```python
from build123d import *

# Parameters (mm, degrees)
SKETCH1_W           = 9.4
SKETCH1_H           = 2
BOSS_EXTRUDE1_DEPTH = 85.5
BOSS_EXTRUDE2_DEPTH = 81
FILLET1_R           = 0.5
BOSS_EXTRUDE3_DEPTH = 78
SKETCH2_R           = 1.5
CUT_EXTRUDE1_DEPTH  = 87.643786319
CUT_EXTRUDE2_REACH  = 88.644
SKETCH2_3_W         = 4.8
SKETCH2_3_H         = 4
SKETCH2_3_W_2       = 2.2
SKETCH3_W           = 2
SKETCH3_H           = 63
CUT_EXTRUDE3_DEPTH  = 5
SKETCH4_W           = 1
SKETCH4_H           = 3.5
CUT_EXTRUDE4_DEPTH  = 2


with BuildPart() as part:
    # Sketch1 → Boss-Extrude1 (new body)
    with BuildSketch(Plane(origin=(0, 0, 0), x_dir=(1, 0, 0), z_dir=(0, 1, 0))):
        with Locations((0.278560628, 2.818575451)):
            Rectangle(SKETCH1_W, SKETCH1_H)
    extrude(amount=-BOSS_EXTRUDE1_DEPTH)

    # Sketch1<3> → Boss-Extrude2 (add)
    with BuildSketch(Plane(origin=(0, 0, 0), x_dir=(1, 0, 0), z_dir=(0, 1, 0))):
        Polygon((3.978560628, 1.818575451), (-3.421439372, 1.818575451), (-3.421439372, 0.818575451), (-4.421439372, 0.818575451), (-4.421439372, -0.181424549), (4.978560628, -0.181424549), (4.978560628, 0.818575451), (3.978560628, 0.818575451), align=None)
    extrude(amount=-BOSS_EXTRUDE2_DEPTH)

    # Fillet1
    fillet1_edges = [part.edges().sort_by_distance(p)[0] for p in [
        (-4.421439372, -85.5, -2.818575451),
        (4.978560628, -85.5, -2.818575451),
        (-4.421439372, 0, -2.818575451),
        (0.278560628, 0, -3.818575451),
        (4.978560628, 0, -2.818575451),
        (-4.421439372, -42.75, -3.818575451),
        (4.978560628, -42.75, -3.818575451),
        (0.278560628, -85.5, -3.818575451),
    ]]
    fillet(fillet1_edges, radius=FILLET1_R)

    # Sketch1<4> → Boss-Extrude3 (add)
    with BuildSketch(Plane(origin=(0, 0, 0), x_dir=(1, 0, 0), z_dir=(0, 1, 0))):
        Polygon((-5.421439372, -0.181424549), (-4.421439372, -0.181424549), (4.978560628, -0.181424549), (5.978560628, -0.181424549), (5.978560628, -8.181424549), (2.978560628, -8.181424549), (2.978560628, -3.181424549), (-4.050977977, -3.181424549), (-4.050977977, -1.181424549), (-5.421439372, -1.181424549), align=None)
    extrude(amount=-BOSS_EXTRUDE3_DEPTH)

    # Sketch2 → Cut-Extrude1 (cut, through all)
    with BuildSketch(Plane(origin=(5.978560628, 0, 0), x_dir=(0, 0, -1), z_dir=(1, 0, 0))):
        with Locations((-5.681424549, -12.5)):
            Circle(SKETCH2_R)
        with Locations((-4.181424549, -75)):
            Circle(SKETCH2_R)
    extrude(amount=-CUT_EXTRUDE1_DEPTH, mode=Mode.SUBTRACT)

    # Cut-Extrude2: up to this face of the body (flat: up to its plane)
    cut_extrude2_end = Plane(part.part.faces().sort_by_distance((3.978560628, -40.5, -1.318575451))[0])
    # Sketch2<3> → Cut-Extrude2 (cut, up to the picked face)
    with BuildSketch(Plane(origin=(5.978560628, 0, 0), x_dir=(0, 0, -1), z_dir=(1, 0, 0)), mode=Mode.PRIVATE) as cut_extrude2_sk1:
        with Locations((-2.581424549, -7)):
            Rectangle(SKETCH2_3_W, SKETCH2_3_H)
    cut_extrude2_tool1 = split(extrude(cut_extrude2_sk1.sketch, amount=-CUT_EXTRUDE2_REACH, mode=Mode.PRIVATE), bisect_by=cut_extrude2_end, keep=Keep.BOTH, mode=Mode.PRIVATE)
    # Sketch2<3> → Cut-Extrude2 (cut, up to the picked face)
    with BuildSketch(Plane(origin=(5.978560628, 0, 0), x_dir=(0, 0, -1), z_dir=(1, 0, 0)), mode=Mode.PRIVATE) as cut_extrude2_sk2:
        with Locations((0.918575451, -7)):
            Rectangle(SKETCH2_3_W_2, SKETCH2_3_H)
    cut_extrude2_tool2 = split(extrude(cut_extrude2_sk2.sketch, amount=-CUT_EXTRUDE2_REACH, mode=Mode.PRIVATE), bisect_by=cut_extrude2_end, keep=Keep.BOTH, mode=Mode.PRIVATE)
    add(cut_extrude2_tool1.solids().sort_by(Axis((5.978561, -7, 2.581425), (-1, 0, 0)))[0], mode=Mode.SUBTRACT)
    add(cut_extrude2_tool2.solids().sort_by(Axis((5.978561, -7, -0.918575), (-1, 0, 0)))[0], mode=Mode.SUBTRACT)

    # Sketch3 → Cut-Extrude3 (cut)
    with BuildSketch(Plane.XY.offset(8.181424549)):
        with Locations((3.978560628, -46.5)):
            Rectangle(SKETCH3_W, SKETCH3_H)
    extrude(amount=-CUT_EXTRUDE3_DEPTH, mode=Mode.SUBTRACT)

    # Sketch4 → Cut-Extrude4 (cut)
    with BuildSketch(Plane(origin=(5.978560628, 0, 0), x_dir=(0, 0, -1), z_dir=(1, 0, 0))):
        with Locations((-2.681424549, -26.75)):
            Rectangle(SKETCH4_W, SKETCH4_H)
        with Locations((-2.681424549, -56.25)):
            Rectangle(SKETCH4_W, SKETCH4_H)
    extrude(amount=-CUT_EXTRUDE4_DEPTH, mode=Mode.SUBTRACT)


with BuildPart() as body_2:
    # Mirror1: mirrored copy
    add(part.part.mirror(Plane(origin=(0, 0, -13.818575451), x_dir=(1, 0, 0), z_dir=(0, 0, -1))))


solid = body_2.part
```
Part model, mm, in its own coordinate system. A direction names the side the tool comes from. Round coordinates to 2 decimals unless told otherwise and drop trailing zeros. Order: outer loops, then holes, each group sorted by start corner. A loop starts at its lowest first (then second) coordinate and runs counter-clockwise, first axis right, second up. Notation, with made-up numbers: M 65,27 L 72,27 A37 cw 72,64 Z; hole C -16,7.25 d8. An arc over 180 degrees is marked long. Answer in a Markdown table with one row per item. Add a question column.
Q1. Wall check: L1, parallel to Z at x = -4, y = -9.5; L2, parallel to Y at x = 1.5, z = -29.5; L3, parallel to X at y = -53, z = -34. Give the ranges that are in metal, low to high. Write a range as from..to.
Q2. Cut at C-C on y = -63.5. Give the cut face in (x, z).
Q3. Cut at A-A on y = -12.5. Give the cut face in (x, z).
Q4. 3-axis set-ups, long thin cutter, end or side, ignore diameter. For faces 5 (the face through (4, -15, -33)), 6 (the face through (-4, -52, -25.819)), 7 (the face through (0, -79, -27.819)): which of +Z, -Z, +X, -X, +Y, -Y reach the whole face in a straight line?
Q5. Pin check, flat tips, straight feed: pin 1 (0.8 mm diameter, centred on y = -55, z = -25, fed in from -X); pin 2 (0.8 mm diameter, centred on x = 5.5, y = -55.5, fed in from +Z); pin 3 (0.5 mm diameter, centred on x = 5.5, z = -30.5, fed in from -Y). Stop position of each tip, or through.
Q6. Mould opens along Z. For faces 1 (the face through (5, -7, -32.619)), 2 (the face through (1, -77, -30.819)), 3 (the face through (0, -42, -23.819)), 4 (the face through (-4.421, -42, -25)) say: +Z half, -Z half, draft (parallel to the pull), parting line (faces both ways), or undercut.
Q7. Cut at B-B on x = 1.5. Give the cut face in (y, z).
Established:
| question | item | result |
|---|---|---|
| 1 | L1 | z = -30.82..-26.82, -25.82..-23.82 |
| 1 | L2 | y = -78..0 |
| 1 | L3 | x = 4.98..5.98 |
| 2 | outline | M -5.42,-28.82 L -4.05,-28.82 L -4.05,-30.82 L 4.98,-30.82 L 4.98,-35.82 L 5.98,-35.82 L 5.98,-27.82 L 4.98,-27.82 L 4.98,-26.82 L 3.98,-26.82 L 3.98,-25.82 L 4.98,-25.82 L 4.98,-24.32 A0.5 ccw 4.48,-23.82 L -3.92,-23.82 A0.5 ccw -4.42,-24.32 L -4.42,-25.82 L -3.42,-25.82 L -3.42,-26.82 L -4.42,-26.82 L -4.42,-27.82 L -5.42,-27.82 Z |
| 3 | outline | M -5.42,-28.82 L -4.05,-28.82 L -4.05,-30.82 L 2.98,-30.82 L 2.98,-31.82 L 5.98,-31.82 L 5.98,-27.82 L 4.98,-27.82 L 4.98,-26.82 L 3.98,-26.82 L 3.98,-25.82 L 4.98,-25.82 L 4.98,-24.32 A0.5 ccw 4.48,-23.82 L -3.92,-23.82 A0.5 ccw -4.42,-24.32 L -4.42,-25.82 L -3.42,-25.82 L -3.42,-26.82 L -4.42,-26.82 L -4.42,-27.82 L -5.42,-27.82 Z; M 2.98,-35.82 L 5.98,-35.82 L 5.98,-34.82 L 2.98,-34.82 Z |
| 4 | face 5 | -Z, -X, -Y |
| 4 | face 6 | -Y |
| 4 | face 7 | -Z, +X, -X, -Y |
| 5 | pin 1 | stops at x = -4.42 |
| 5 | pin 2 | stops at z = -27.82 |
| 5 | pin 3 | stops at y = -78 |
| 6 | face 1 | undercut |
| 6 | face 2 | -Z half |
| 6 | face 3 | +Z half |
| 6 | face 4 | draft |
| 7 | outline | M -85.5,-25.82 L -81,-25.82 L -81,-27.82 L -78,-27.82 L -78,-30.82 L -76.12,-30.82 A1.5 cw -73.88,-30.82 L 0,-30.82 L 0,-24.32 A0.5 ccw -0.5,-23.82 L -85,-23.82 A0.5 ccw -85.5,-24.32 Z |
